from build123d import *

# Parameters (mm, degrees)
F0_W     = 10.1
F0_H     = 12.5
F0_W_2   = 6.1
F0_H_2   = 8.5
F1_DEPTH = 15
F3_DEPTH = 1.5
F5_DEPTH = 24.3923048454
F7_DEPTH = 25


with BuildPart() as f1:
    # F0 (on Right) → F1 (new body)
    with BuildSketch(Plane.YZ):
        Rectangle(F0_W, F0_H)
        Rectangle(F0_W_2, F0_H_2, mode=Mode.SUBTRACT)
    extrude(amount=F1_DEPTH)

    # F2 (on Front) → F3 (join, symmetric)
    with BuildSketch(Plane.XZ):
        Polygon((-5.1961524227, 9.25), (0, 6.25), (14, 6.25), (19.1961524227, 9.25), (19.1961524227, 11.25), (-5.1961524227, 11.25), align=None)
    extrude(amount=F3_DEPTH, both=True)

    # F4 (on face) → F5 (join, through all)
    with BuildSketch(Plane(origin=(-5.1961524227, 0, 0), x_dir=(0, -1, 0), z_dir=(-1, 0, 0))):
        Polygon((15, 15.2692378865), (0, 11.25), (1.5, 9.25), (15, 13.2692378865), align=None)
        Polygon((-1.5, 9.25), (0, 11.25), (-15, 15.2692378865), (-15, 13.2692378865), align=None)
    extrude(amount=-F5_DEPTH)

    # F6 (on Top) → F7 (cut)
    with BuildSketch(Plane.XY):
        Polygon((14.1379434391, 18.8774929223), (19.1961524227, 0), (14.1379434391, -18.8774929223), (27.2481460124, -18.8774929223), (27.2481460124, 0), (27.2481460124, 18.8774929223), align=None)
    extrude(amount=F7_DEPTH, mode=Mode.SUBTRACT)


solid = f1.part
Could you check a few things on this model? Use its own coordinates, in mm. A direction names the side the tool comes from. Give positions to 0.01 mm unless a question says otherwise; leave off trailing zeros. Write each loop counter-clockwise with the first axis right and the second up, starting at its lowest first coordinate (ties: lowest second). Pieces come first, ordered by that corner, then holes. Notation, with made-up numbers: (55, -4.75) -> (113, -4.75) arc R28 cw to (113, 16.25) -> close; hole circle Ø10 at (-14.75, 67.25). An arc over 180 degrees is marked (long way). Write each question's results on one line, items separated by ' | '. Start each with the question number.
Q1. Suppose I cut it at D-D, the plane y = 9. List the corners of the cut face in (x, z) for me.
Q2. Suppose I cut it at C-C, the plane z = 4.75. List the corners of the cut face in (x, y) for me.
Q3. Which directions (+Z, -Z, +X, -X, +Y, -Y) give clear straight access to the entire face, cutting with the end or side of a thin tool? Please do faces 1 (the face through (7, 5.05, 0)), 2 (the face through (15, -3.4, 0.1)), 3 (the face through (7, 3.05, 0)), 4 (the face through (7, -5.05, 0)), 5 (the face through (6.631, -8.156, 11.231)).
Q4. We'd pull the mould along Z, two halves only. Please class faces 6 (the face through (-2.63, -0.02, 7.77)), 7 (the face through (6.829, -7.605, 13.288)), 8 (the face through (17.196, -7.465, 11.897)), 9 (the face through (7, 0, 4.25)): +Z half, -Z half, draft (parallel to the pull), parting line (faces both ways), or undercut.
Q5. I'm going to push flat-ended pins straight in: pin 1 Ø5 at (y, z) = (12, 9.5) entering from +X; pin 2 Ø4 at (x, z) = (5, 0.5) entering from -Y; pin 3 Ø0.9 at (x, z) = (8, 8.5) entering from +Y; pin 4 Ø6 at (x, z) = (9, -0.5) entering from +Y. Where does each tip first touch, or does it pass through?
Q6. Suppose I cut it at B-B, the plane x = 0.75. List the corners of the cut face in (y, z) for me, and give its area (3 significant figures).
Q7. I need wall thicknesses on probe 1 along Y at (x, z) = (1.75, 3.75); probe 2 along Z at (x, y) = (2.75, -3); probe 3 along Z at (x, y) = (4, -2.5). Which ranges of each line are inside material? Lowest first, please.
Q8. Suppose I cut it at A-A, the plane z = 0.5. List the corners of the cut face in (x, y) for me, and give its area (3 significant figures).
Outcome:
1) outline: (-5.2, 11.48) -> (16.78, 11.48) -> (16.78, 13.66) -> (-5.2, 13.66) -> close
2) outline: (0, -5.05) -> (15, -5.05) -> (15, 5.05) -> (0, 5.05) -> close
3) face 1: -Z, +X, -X, +Y | face 2: -Z, +X, +Y, -Y | face 3: +X, -X | face 4: -Z, +X, -X, -Y | face 5: +X, -X, -Y
4) face 6: -Z half | face 7: +Z half | face 8: draft | face 9: undercut
5) pin 1: through | pin 2: y = -5.05 | pin 3: y = 1.5 | pin 4: y = 5.05
6) outline: (-15, 13.27) -> (-1.5, 9.25) -> (-1.5, 6.25) -> (-5.05, 6.25) -> (-5.05, -6.25) -> (5.05, -6.25) -> (5.05, 6.25) -> (1.5, 6.25) -> (1.5, 9.25) -> (15, 13.27) -> (15, 15.27) -> (0, 11.25) -> (-15, 15.27) -> close; hole (-3.05, -4.25) -> (3.05, -4.25) -> (3.05, 4.25) -> (-3.05, 4.25) -> close | area: 149 mm2
7) probe 1: -5.05 to -3.05, 3.05 to 5.05 | probe 2: -6.25 to -4.25, 4.25 to 6.25, 9.7 to 12.05 | probe 3: -6.25 to -4.25, 4.25 to 6.25, 9.55 to 11.92
8) outline: (0, -5.05) -> (15, -5.05) -> (15, -3.05) -> (0, -3.05) -> close; (0, 3.05) -> (15, 3.05) -> (15, 5.05) -> (0, 5.05) -> close | area: 60.0 mm2
